The model under review builds one solid part; all positions refer to its coordinate system, in mm. A direction names the side the tool comes from. Give positions to 0.01 mm unless a question says otherwise; leave off trailing zeros. Write each loop counter-clockwise with the first axis right and the second up, starting at its lowest first coordinate (ties: lowest second). Pieces come first, ordered by that corner, then holes. Notation, with made-up numbers: M 76.5,-28.5 L 115.5,-28.5 A37 cw 115.5,9.5 Z; hole C -16,-27.75 d1. An arc over 180 degrees is marked long. Write item = value, one per line. Start each with the question number.
```python
from build123d import *

# Parameters (mm, degrees)
F1_DEPTH = 20
F3_D     = 6.2484
F5_W     = 45
F5_H     = 5.25
F5_H_2   = 6.15
F6_DEPTH = 5
F4_W     = 45
F4_H     = 5.25
F4_H_2   = 6.15
F7_DEPTH = 5
F8_R     = 5
F9_R     = 2.193764509
F11_D    = 9
F13_D    = 5


with BuildPart() as f1:
    # F0 (on Top) → F1 (new body)
    with BuildSketch(Plane.XY):
        Polygon((80, 0), (0, 0), (0, -6), (74, -6), (74, -51), (156, -51), (156, 0), (150, 0), (150, -45), (80, -45), align=None)
    extrude(amount=F1_DEPTH)

    # F3 (through all)
    with Locations(Plane(origin=(0, 0, 0), x_dir=(-1, 0, 0), z_dir=(0, 1, 0))):
        with Locations((-45, 10), (-30, 10), (-15, 10)):
            Hole(F3_D / 2)

    # F5 (on face) → F6 (join)
    with BuildSketch(Plane(origin=(150, 0, 0), x_dir=(0, -1, 0), z_dir=(-1, 0, 0))):
        with Locations((22.5, 17.375)):
            Rectangle(F5_W, F5_H)
        with Locations((22.5, 3.075)):
            Rectangle(F5_W, F5_H_2)
    extrude(amount=F6_DEPTH)

    # F4 (on face) → F7 (join)
    with BuildSketch(Plane.YZ.offset(80)):
        with Locations((-22.5, 17.375)):
            Rectangle(F4_W, F4_H)
        with Locations((-22.5, 3.075)):
            Rectangle(F4_W, F4_H_2)
    extrude(amount=F7_DEPTH)

    # F8
    f8_edges = [f1.edges().sort_by_distance(p)[0] for p in [
        (74, -51, 10),
        (156, -51, 10),
        (0, 0, 10),
    ]]
    fillet(f8_edges, radius=F8_R)

    # F9
    f9_edges = [f1.edges().sort_by_distance(p)[0] for p in [
        (85, -22.5, 14.75),
        (145, -22.5, 14.75),
    ]]
    fillet(f9_edges, radius=F9_R)

    # F11 (through all)
    with Locations(Plane.XZ.offset(51)):
        with Locations((115, 10)):
            Hole(F11_D / 2)

    # F13 (through all)
    with Locations(Plane.YZ.offset(156)):
        with Locations((-23, 10)):
            Hole(F13_D / 2)


solid = f1.part
```
Item 1: For faces 5 (the cylindrical face through (14.6, -3, 13.1)), 6 (the flat face through (145, -22, 3)), 7 (the flat face through (82, -23, 6.15)), 8 (the flat face through (44, 0, 14)), 9 (the flat face through (36, -6, 10)), list the 3-axis set-ups (+Z, -Z, +X, -X, +Y, -Y) from which the entire face can be reached by the end or side of a thin tool; tool diameter is ignored.
Item 2: Clearance check with flat-ended pins moving along their axes: P1, Ø2, axis at y = -45, z = 15.5, coming from the -X side; P2, Ø3, axis at x = 148.5, y = -22, coming from the -Z side; P3, Ø10, axis at x = 30, z = 10, coming from the -Y side. State where each tip first meets the part, or that it passes through.
Item 3: The part is to be moulded in two halves that separate along Z. For faces 1 (the flat face through (83, -25, 0)), 2 (the flat face through (84, -23, 20)), 3 (the cylindrical face through (1, -2, 10)), 4 (the flat face through (149, -22, 14.75)), say which applies: released by +Z, released by -Z, zero draft, split by the parting line, or undercut.
Item 4: We need section C-C, the plane z = 2.25. Write out the cut boundary in (x, y), and give its area (3 significant figures).
Item 5: To check wall thickness, follow probe 1 along X at (y, z) = (-32, 6); probe 2 along X at (y, z) = (-5.5, 13.5); probe 3 along Z at (x, y) = (148, -12.5). State the ranges of each line that lie inside material, in increasing order. Write a range as [from, to].
Item 6: We need section A-A, the plane y = -40.5. Write out the cut boundary in (x, z), and give its area (3 significant figures).
Item 7: We need section B-B, the plane x = 30. Write out the cut boundary in (y, z).
Item 8: We need section D-D, the plane y = -23. Write out the cut boundary in (x, z), and give its area (3 significant figures).
Worked out:
q1.face_5 = +Y, -Y
q1.face_6 = +Z, -Z, +Y
q1.face_7 = +Y
q1.face_8 = +Z, -Z, +X, -X, +Y
q1.face_9 = +Z, -Z, -X, -Y
q2.P1 = 74
q2.P2 = 0
q2.P3 = -6
q3.face_1 = released by -Z
q3.face_2 = released by +Z
q3.face_3 = zero draft
q3.face_4 = undercut
q4.outline = M 0,-6 L 74,-6 L 74,-46 A5 ccw 79,-51 L 151,-51 A5 ccw 156,-46 L 156,0 L 145,0 L 145,-45 L 85,-45 L 85,0 L 5,0 A5 ccw 0,-5 Z
q4.area = 1,910 mm²
q5.probe_1 = [74, 85], [145, 156]
q5.probe_2 = [0, 80], [150, 156]
q5.probe_3 = [0, 6.15], [14.75, 20]
q6.outline = M 74,0 L 85,0 L 85,6.15 L 80,6.15 L 80,14.75 L 82.81,14.75 A2.19 ccw 85,16.94 L 85,20 L 74,20 Z; M 145,0 L 156,0 L 156,20 L 145,20 L 145,16.94 A2.19 ccw 147.19,14.75 L 150,14.75 L 150,6.15 L 145,6.15 Z
q6.area = 352 mm²
q7.outline = M -6,0 L 0,0 L 0,6.88 L -6,6.88 Z; M -6,13.12 L 0,13.12 L 0,20 L -6,20 Z
q8.outline = M 74,0 L 85,0 L 85,6.15 L 80,6.15 L 80,7.5 L 74,7.5 Z; M 74,12.5 L 80,12.5 L 80,14.75 L 82.81,14.75 A2.19 ccw 85,16.94 L 85,20 L 74,20 Z; M 145,0 L 156,0 L 156,7.5 L 150,7.5 L 150,6.15 L 145,6.15 Z; M 145,16.94 A2.19 ccw 147.19,14.75 L 150,14.75 L 150,12.5 L 156,12.5 L 156,20 L 145,20 Z
q8.area = 292 mm²
